Work out the finished part from the listing and answer in its coordinate system (mm). Coordinates: 2 decimals unless noted, no trailing zeros. Write each loop counter-clockwise with the first axis right and the second up, starting at its lowest first coordinate (ties: lowest second). Pieces come first, ordered by that corner, then holes. Notation, with made-up numbers: (-3.75, -30) -> (47.25, -30) arc R32 ccw to (47.25, 0) -> close; hole circle Ø1 at (69.25, -39.5). An arc over 180 degrees is marked (long way). Write each question's results on one line, items separated by ' | '. Start each with the question number.
from build123d import *

# Parameters (mm, degrees)
F0_R     = 5
F1_DEPTH = 10


with BuildPart() as f1:
    # F0 (on Front) → F1 (new body)
    with BuildSketch(Plane.XZ):
        with BuildLine():
            ThreePointArc((0, 50), (-35.355339, -35.355339), (50, 0))
            ThreePointArc((50, 0), (35.355339, 35.355339), (0, 50))
        make_face()
        with Locations((-28.284271, -28.284271)):
            Circle(F0_R, mode=Mode.SUBTRACT)
        with Locations((0, -40)):
            Circle(F0_R, mode=Mode.SUBTRACT)
        with Locations((28.284271, -28.284271)):
            Circle(F0_R, mode=Mode.SUBTRACT)
        with Locations((-40, 0)):
            Circle(F0_R, mode=Mode.SUBTRACT)
        with Locations((-28.284271, 28.284271)):
            Circle(F0_R, mode=Mode.SUBTRACT)
        with BuildLine():
            ThreePointArc((30, 0), (-21.213203, -21.213203), (0, 30))
            ThreePointArc((0, 30), (21.213203, 21.213203), (30, 0))
        make_face(mode=Mode.SUBTRACT)
        with Locations((40, 0)):
            Circle(F0_R, mode=Mode.SUBTRACT)
        with BuildLine():
            ThreePointArc((0, 35), (-5, 40), (0, 45))
            ThreePointArc((0, 45), (3.535534, 43.535534), (5, 40))
            ThreePointArc((5, 40), (3.535534, 36.464466), (0, 35))
        make_face(mode=Mode.SUBTRACT)
        with Locations((28.284271, 28.284271)):
            Circle(F0_R, mode=Mode.SUBTRACT)
    extrude(amount=F1_DEPTH)


solid = f1.part
1. Given pin 1 Ø1 at (x, y) = (6, -1.5) entering from -Z; pin 2 Ø1 at (x, y) = (-4, -9) entering from -Z; pin 3 Ø1 at (y, z) = (-7, 21) entering from +X, each flat-ended and moving along its own axis, determine where each tip first touches the part or whether it passes through.
2. Determine the mould class of faces 1 (the face through (22, -10, -22)), 2 (the face through (24.32, -4.93, 25.24)) for opening direction X: pulls with the +X half, pulls with the -X half, needs draft (parallel to the pull), parting line crosses it, or undercut.
3. Find section C-C on x = 32. Give the vertices of the cut face in (y, z), and give its area (3 significant figures).
4. Find section B-B on z = -40. Give the vertices of the cut face in (x, y), and give its area (3 significant figures).
5. Find the intervals of material crossed by L1, parallel to Z at x = -26.5, y = -7.5; L2, parallel to Z at x = -1.5, y = -6.5; L3, parallel to Z at x = -40, y = -5.75, in increasing order.
6. Find section A-A on x = -40. Give the vertices of the cut face in (y, z), and give its area (3 significant figures).
7. Find section D-D on z = 27. Give the vertices of the cut face in (x, y), and give its area (3 significant figures).
Ans:
1) pin 1: stops at z = -49.7 | pin 2: stops at z = -49.88 | pin 3: stops at x = 45.6
2) face 1: needs draft | face 2: undercut
3) outline: (-10, -38.42) -> (0, -38.42) -> (0, -31.63) -> (-10, -31.63) -> close; (-10, -24.94) -> (0, -24.94) -> (0, 24.94) -> (-10, 24.94) -> close; (-10, 31.63) -> (0, 31.63) -> (0, 38.42) -> (-10, 38.42) -> close | area: 635 mm²
4) outline: (-30, -10) -> (-5, -10) -> (-5, 0) -> (-30, 0) -> close; (5, -10) -> (30, -10) -> (30, 0) -> (5, 0) -> close | area: 500 mm²
5) L1: z = -42.4 to -32.96, -23.61 to -14.06, 14.06 to 23.61, 32.96 to 42.4 | L2: z = -49.98 to -44.77, -35.23 to -29.96, 29.96 to 35.23, 44.77 to 49.98 | L3: z = -30 to -5, 5 to 30
6) outline: (-10, -30) -> (0, -30) -> (0, -5) -> (-10, -5) -> close; (-10, 5) -> (0, 5) -> (0, 30) -> (-10, 30) -> close | area: 500 mm²
7) outline: (-42.08, -10) -> (-33.12, -10) -> (-33.12, 0) -> (-42.08, 0) -> close; (-23.45, -10) -> (-13.08, -10) -> (-13.08, 0) -> (-23.45, 0) -> close; (13.08, -10) -> (23.45, -10) -> (23.45, 0) -> (13.08, 0) -> close; (33.12, -10) -> (42.08, -10) -> (42.08, 0) -> (33.12, 0) -> close | area: 387 mm²
